Geometry check sheet. Reference: the model listing, model coordinates, mm. A direction names the side the tool comes from. Give positions to 0.01 mm unless a question says otherwise; leave off trailing zeros. Order: outer loops, then holes, each group sorted by start corner. A loop starts at its lowest first (then second) coordinate and runs counter-clockwise, first axis right, second up. Notation, with made-up numbers: (51, 52.5) - (110, 52.5) arc R30 cw to (110, 77.5) - close; hole circle Ø1 at (-22.75, -30). An arc over 180 degrees is marked (long way). Put each result on its own line as item: value. Start each with the question number.
```python
from build123d import *

# Parameters (mm, degrees)
F0_W     = 76.2
F0_H     = 25.4
F1_DEPTH = 25.4
F2_W     = 25.4508
F2_H     = 12.7254
F3_DEPTH = 25.4
F4_W     = 12.7254
F4_H     = 12.7254
F5_DEPTH = 25.654
F6_W     = 12.6873
F6_H     = 12.7
F7_DEPTH = 25.654
F9_DEPTH = 25.4


with BuildPart() as f1:
    # F0 (on Top) → F1 (new body)
    with BuildSketch(Plane.XY):
        with Locations((38.1, 12.7)):
            Rectangle(F0_W, F0_H)
    extrude(amount=F1_DEPTH)

    # F2 (on Front) → F3 (cut)
    with BuildSketch(Plane.XZ):
        with Locations((38.1, 19.4584317505)):
            Rectangle(F2_W, F2_H)
    extrude(amount=-F3_DEPTH, mode=Mode.SUBTRACT)

    # F4 (on face) → F5 (cut)
    with BuildSketch(Plane.XY.offset(25.4)):
        with Locations((19.0119, 6.3627)):
            Rectangle(F4_W, F4_H)
    extrude(amount=-F5_DEPTH, mode=Mode.SUBTRACT)

    # F6 (on face) → F7 (cut)
    with BuildSketch(Plane.XY.offset(25.4)):
        with Locations((57.16905, 6.35)):
            Rectangle(F6_W, F6_H)
    extrude(amount=-F7_DEPTH, mode=Mode.SUBTRACT)

    # F8 (on face) → F9 (cut)
    with BuildSketch(Plane.XY.offset(13.0957317505)):
        Polygon((38.1, 0), (50.8254, 0), (50.8254, 12.7), (50.8254, 12.7254), (38.1, 12.7254), align=None)
    extrude(amount=-F9_DEPTH, mode=Mode.SUBTRACT)


solid = f1.part
```
Item 1: Gauge pin test, flat end, axial feed: pin 1 Ø4 at (x, z) = (59.5, 12.5) entering from -Y. Record the tip position at first contact, or that the pin passes through.
Item 2: Cross-section at B-B (z = 21.25). Enter the section's corners in (x, y), and give its area (3 significant figures).
Item 3: Cross-section at C-C (y = 22.25). Enter the section's corners in (x, z), and give its area (3 significant figures).
Item 4: Thickness scan on line 1 along X through (y, z) = (9.75, 11.25); line 2 along X through (y, z) = (13.5, 21); line 3 along Z through (x, y) = (25.5, 8.75). Record the ranges inside material, lowest first.
Item 5: Set-up check for faces 4 (the face through (45, 12.725, 7)), 5 (the face through (6, 0, 13)), 6 (the face through (25.375, 19, 19)): record each of +Z, -Z, +X, -X, +Y, -Y from which the full face is reachable in a straight line by a thin tool's end or side.
Item 6: Cross-section at A-A (y = 11.25). Enter the section's corners in (x, z), and give its area (3 significant figures).
Item 7: Release check for a two-part mould opening along X. For faces 1 (the face through (63.513, 6, 13)), 2 (the face through (10, 16, 25.4)), 3 (the face through (76.2, 13, 13)) record: +X half, -X half, draft (parallel to the pull), parting line (faces both ways), or undercut.
Recorded:
1. pin 1: stops at y = 12.7
2. outline: (0, 0) - (12.65, 0) - (12.65, 12.73) - (25.37, 12.73) - (25.37, 25.4) - (0, 25.4) - close; (50.83, 12.7) - (63.51, 12.7) - (63.51, 0) - (76.2, 0) - (76.2, 25.4) - (50.83, 25.4) - close
2. area: 966 mm^2
3. outline: (0, 0) - (76.2, 0) - (76.2, 25.4) - (50.83, 25.4) - (50.83, 13.1) - (25.37, 13.1) - (25.37, 25.4) - (0, 25.4) - close
3. area: 1,620 mm^2
4. line 1: x = 0 to 12.65, 25.37 to 38.1, 63.51 to 76.2
4. line 2: x = 0 to 25.37, 50.83 to 76.2
4. line 3: z = 0 to 13.1
5. face 4: +Z, -Z, -Y
5. face 5: +Z, -Z, +X, -X, -Y
5. face 6: +Z, +Y, -Y
6. outline: (0, 0) - (12.65, 0) - (12.65, 25.4) - (0, 25.4) - close; (25.37, 0) - (38.1, 0) - (38.1, 13.1) - (25.37, 13.1) - close; (63.51, 0) - (76.2, 0) - (76.2, 25.4) - (63.51, 25.4) - close
6. area: 810 mm^2
7. face 1: undercut
7. face 2: draft
7. face 3: +X half
